Can you work these out from the model? Positions are in its coordinate system, mm. Face numbers are marked on the shaded views. A direction names the side the tool comes from. Round coordinates to 2 decimals unless told otherwise and drop trailing zeros. Write each loop counter-clockwise with the first axis right and the second up, starting at its lowest first coordinate (ties: lowest second). Pieces come first, ordered by that corner, then holes. Notation, with made-up numbers: (-16, 22.25) - (18, 22.25) arc R28 ccw to (18, 48.25) - close; hole circle Ø4 at (80.25, 83.25). An arc over 180 degrees is marked (long way). One line per item, written item: value. Start each with the question number.
(1) On a 3-axis mill with a long thin cutter (end or side, diameter ignored), from which of +Z, -Z, +X, -X, +Y, -Y can I reach the whole of each face in a straight line? I mean the marked faces 4 and 5. Say none if no direction works.
(2) If I drill on L1, parallel to Y at x = 0, z = 8; L2, parallel to Z at x = -24.5, y = 3.5; L3, parallel to X at y = -7, z = 7, over which ranges is the centre line in solid material (lowest first)? Write a range as from..to.
(3) I want a section at D-D on x = 6.5. List the corners of the cut face in (y, z) for me, plus the area to 3 significant figures.
(4) Thinking about a two-plate mould opening in Y: for the marked faces 1, 2 and 3, which applies, +Y half, -Y half, draft (parallel to the pull), parting line (faces both ways), or undercut?
(5) I want a section at C-C on z = 12.5. List the corners of the cut face in (x, y) for me.
(6) I want a section at B-B on y = 0. List the corners of the cut face in (x, z) for me (3 decimals), plus the area to 3 significant figures.
(7) I want a section at A-A on x = 0. List the corners of the cut face in (y, z) for me (3 decimals).
(8) I'm going to push flat-ended pins straight in: pin 1 Ø12 at (x, y) = (14.5, -11) entering from -Z; pin 2 Ø10 at (y, z) = (6.5, 19.5) entering from -X; pin 3 Ø4 at (x, y) = (13.5, 14.5) entering from +Z; pin 4 Ø1.6 at (x, z) = (0, 16.5) entering from -Y. Where does each tip first touch, or does it pass through?
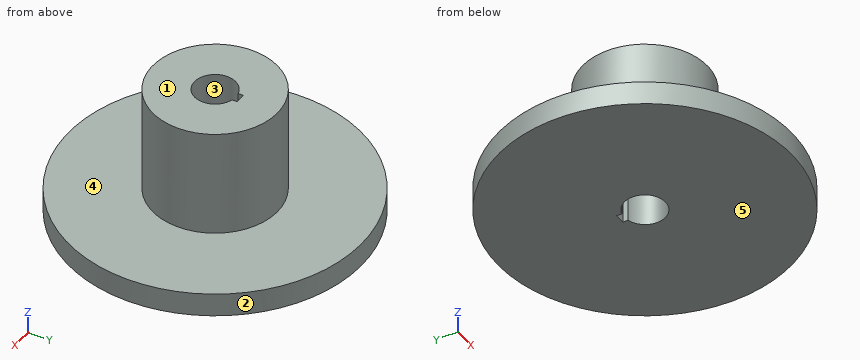
Autodesk Inventor part; units mm, degrees
ref_plane "YZ Plane" through (0, 0, 0) normal (1, 0, 0) x (0, 1, 0)
ref_plane "XZ Plane" through (0, 0, 0) normal (0, 1, 0) x (-1, 0, 0)
ref_plane "XY Plane" through (0, 0, 0) normal (0, 0, 1) x (1, 0, 0)
sketch "Sketch1" plane through (0, 0, 0) normal (0, 0, 1) x (1, 0, 0)
  circle A0 centre (0, 0) radius 28.575
  dimension "d0" = 57.15
extrude "Extrusion1" add sketch "Sketch1" along normal blind 4.572
sketch "Sketch2" plane through (0, 0, 4.572) normal (0, 0, 1) x (1, 0, 0)
  circle A0 centre (0, 0) radius 28.575
  circle A1 centre (0, 0) radius 12.1666
  dimension "d3" = 24.3332
extrude "Extrusion2" add sketch "Sketch2" along normal blind 20.828 contours A1
sketch "Sketch3" plane through (0, 0, 25.4) normal (0, 0, 1) x (1, 0, 0)
  circle A0 centre (0, 0) radius 12.1666
  circle A1 centre (0, 0) radius 4
  line L0 (-1, 4.873) -> (1, 4.873)
  line L1 (1, 4.873) -> (1, 2.873)
  line L2 (1, 2.873) -> (-1, 2.873)
  line L3 (-1, 2.873) -> (-1, 4.873)
  point P0 (0, 4.873)
  point P1 (-1, 3.873)
  dimension "d6" = 8
  dimension "d7" = 2
  dimension "d8" = 2
extrude "Extrusion3" cut sketch "Sketch3" against normal through all contours A1 L3 L2 L1 | L1 L2 L3 A1 | A1 L3 L0 L1
properties part number "Hub 8mm key"
Established:
1. face 4: +Z
1. face 5: -Z, +X, -X, +Y, -Y
2. L1: -12.17..-4, 4.87..12.17
2. L2: 0..4.57
2. L3: -9.95..9.95
3. outline: (-27.83, 0) - (27.83, 0) - (27.83, 4.57) - (10.28, 4.57) - (10.28, 25.4) - (-10.28, 25.4) - (-10.28, 4.57) - (-27.83, 4.57) - close
3. area: 683 mm2
4. face 1: draft
4. face 2: parting line
4. face 3: undercut
5. outline: circle Ø24.33 at (0, 0); hole (-1, 3.87) arc R4 ccw (long way) to (1, 3.87) - (1, 4.87) - (-1, 4.87) - close
6. outline: (-28.575, 0) - (-4, 0) - (-4, 25.4) - (-12.167, 25.4) - (-12.167, 4.572) - (-28.575, 4.572) - close; (4, 0) - (28.575, 0) - (28.575, 4.572) - (12.167, 4.572) - (12.167, 25.4) - (4, 25.4) - close
6. area: 565 mm2
7. outline: (-28.575, 0) - (-4, 0) - (-4, 25.4) - (-12.167, 25.4) - (-12.167, 4.572) - (-28.575, 4.572) - close; (4.873, 0) - (28.575, 0) - (28.575, 4.572) - (12.167, 4.572) - (12.167, 25.4) - (4.873, 25.4) - close
8. pin 1: z = 0
8. pin 2: x = -12.07
8. pin 3: z = 4.57
8. pin 4: y = -12.17
